Autodesk Inventor part; units mm, degrees
ref_plane "YZ Plane" through (0, 0, 0) normal (1, 0, 0) x (0, 1, 0)
ref_plane "XZ Plane" through (0, 0, 0) normal (0, 1, 0) x (-1, 0, 0)
ref_plane "XY Plane" through (0, 0, 0) normal (0, 0, 1) x (1, 0, 0)
sketch "Sketch1" plane through (0, 0, 0) normal (0, 0, 1) x (1, 0, 0)
  circle A0 centre (12.7, 635.3302) radius 3.175
  circle A1 centre (12.7, 635.3302) radius 3.175
  circle A2 centre (12.7, 723.9) radius 6.35
  circle A3 centre (12.7, 12.7) radius 6.35
  circle A4 centre (12.7, 368.3) radius 6.35
  line L0 (25.4, 0) -> (0, 0)
  line L1 (0, 0) -> (0, 736.6)
  line L2 (25.4, 736.6) -> (0, 736.6)
  line L3 (25.4, 0) -> (25.4, 736.6)
  line L4 (25.4, 661.652) -> (-101.3077, 653.0401)
  line L5 (-101.3077, 653.0401) -> (-94.4182, 551.6739)
  line L6 (-94.4182, 551.6739) -> (25.4, 559.8176)
  line L7 (25.4, 661.652) -> (25.4, 559.8176)
  circle A5 centre (12.7, 635.3302) radius 3.175
  dimension "d0" = 101.6
  dimension "d1" = 127
  dimension "d2" = 25.4
extrude "Extrusion1" add sketch "Sketch1" along normal blind 6.35 contours L6 L1 L4 L3 | L6 L5 L4 L1
sketch "Sketch2" plane through (0, 0, 0) normal (0, 0, -1) x (-1, 0, 0)
  circle A0 centre (37.4278, 642.601) radius 12.7
  point P0 (0, 0)
extrude "Extrusion2" cut sketch "Sketch2" against normal through all
properties part number "2018 Intake Plate"
Could you check a few things on this model? Use its own coordinates, in mm. Give positions to 0.01 mm unless a question says otherwise; leave off trailing zeros. Loops run counter-clockwise (first coordinate to the right, second up) from the corner with the lowest first, then second, coordinate; pieces in that order, holes last. Notation, with made-up numbers: M 2,84 L 56,84 A24 cw 56,105 Z; hole C 28,10 d10. An arc over 180 degrees is marked long. Answer as a JSON object with one key per item and string values.
Q1. Suppose I cut it at B-B, the plane z = 2.75. List the corners of the cut face in (x, y) for me (3 decimals).
Values found:
{"outline": "M -101.308,653.04 L -94.418,551.674 L 25.4,559.818 L 25.4,661.652 Z; hole C -37.428,642.601 d25.4; hole C 12.7,635.33 d6.35"}
Q2. If we mould it in two halves opening along X, with no side actions, what happens to faces 1 (the flat face through (-39, 607, 6.35)), 2 (the cylindrical face through (14.165, 638.147, 3.131)), 3 (the flat face through (-35.35, 555.69, 3.13))? For each: pulls with the +X half, pulls with the -X half, needs draft (parallel to the pull), parting line crosses it, or undercut.
Values found:
{"face 1": "needs draft", "face 2": "undercut", "face 3": "pulls with the +X half"}
Q3. Suppose I cut it at D-D, the plane x = -74. List the corners of the cut face in (y, z) for me.
Values found:
{"outline": "M 553.06,0 L 654.9,0 L 654.9,6.35 L 553.06,6.35 Z"}
Q4. Suppose I cut it at A-A, the plane x = 12.7. List the corners of the cut face in (y, z) for me, plus the area to 3 significant figures.
Values found:
{"outline": "M 558.95,0 L 632.16,0 L 632.16,6.35 L 558.95,6.35 Z; M 638.51,0 L 660.79,0 L 660.79,6.35 L 638.51,6.35 Z", "area": "606 mm²"}
Q5. If I drill on probe 1 along X at (y, z) = (637.5, 2); probe 2 along Y at (x, z) = (-46, 2.5); probe 3 along Y at (x, z) = (-41.5, 4), over which ranges is the centre line in solid material (lowest first)? Write a range as [from, to].
Values found:
{"probe 1": "x = [-100.25, -49.06], [-25.8, 10.38], [15.02, 25.4]", "probe 2": "y = [554.96, 633.23], [651.97, 656.8]", "probe 3": "y = [555.27, 630.57], [654.63, 657.11]"}
Q6. Suppose I cut it at C-C, the plane y = 571. List the corners of the cut face in (x, z) for me, plus the area to 3 significant figures.
Values found:
{"outline": "M -95.73,0 L 25.4,0 L 25.4,6.35 L -95.73,6.35 Z", "area": "769 mm²"}
Q7. For P1, Ø2, axis at x = 4, z = 2, coming from the +Y side; P2, Ø3, axis at x = -20, z = 2, coming from the -Y side; P3, Ø8.5, axis at x = 12.7, y = 635.33, coming from the -Z side, each with a flat end and sliding along its axis, tell me the tip position at first contact or that it passes through.
Values found:
{"P1": "stops at y = 660.27", "P2": "stops at y = 556.63", "P3": "stops at z = 0"}
